from build123d import *

# Parameters (mm, degrees)
CROQUIS1_W              = 15.2
CROQUIS1_H              = 24.4
CROQUIS1_W_2            = 14
CROQUIS1_H_2            = 6.4
SALIENTE_EXTRUIR2_DEPTH = 8
SALIENTE_EXTRUIR4_START = 5
CROQUIS2_W              = 14
CROQUIS2_H              = 6.4
CROQUIS2_W_2            = 15.2
CROQUIS2_H_2            = 24.4
CROQUIS2_R              = 4
SALIENTE_EXTRUIR4_DEPTH = 5
CROQUIS3_R              = 4
CORTAR_EXTRUIR1_DEPTH   = 25
CROQUIS4_R              = 4
CORTAR_EXTRUIR2_DEPTH   = 30.02
CORTAR_EXTRUIR3_REACH   = 79.24
CROQUIS5_R              = 4.5


with BuildPart() as part:
    # Croquis1 → Saliente-Extruir2 (new body)
    with BuildSketch(Plane.XY):
        with BuildLine():
            Line((9.976185601, 29.499985584), (9.976185601, 16.499985584))
            Line((9.976185601, 16.499985584), (0.021811005, 16.499985584))
            ThreePointArc((0.021811005, 16.499985584), (-16.499996396, 0.010905505), (0, -16.5))
            Line((0, -16.5), (15, -16.5))
            Line((15, -16.5), (15, -29.5))
            Line((15, -29.5), (-14.857693224, -29.5))
            ThreePointArc((-14.857693224, -29.5), (-18.39322713, -28.035533906), (-19.857693224, -24.5))
            Line((-19.857693224, -24.5), (-19.857693224, -21.5))
            ThreePointArc((-19.857693224, -21.5), (-21.322159318, -17.964466094), (-24.857693224, -16.5))
            Line((-24.857693224, -16.5), (-56.53, -16.5))
            ThreePointArc((-56.53, -16.5), (-60.065533906, -15.035533906), (-61.53, -11.5))
            Line((-61.53, -11.5), (-61.53, 11.5))
            ThreePointArc((-61.53, 11.5), (-60.065533906, 15.035533906), (-56.53, 16.5))
            Line((-56.53, 16.5), (-24.857693224, 16.5))
            ThreePointArc((-24.857693224, 16.5), (-21.322159318, 17.964466094), (-19.857693224, 21.5))
            Line((-19.857693224, 21.5), (-19.857693224, 24.499985584))
            ThreePointArc((-19.857693224, 24.499985584), (-18.39322713, 28.03551949), (-14.857693224, 29.499985584))
            Line((-14.857693224, 29.499985584), (9.976185601, 29.499985584))
        make_face()
        with Locations((-49.43, 0)):
            Rectangle(CROQUIS1_W, CROQUIS1_H, mode=Mode.SUBTRACT)
        with Locations((-29, 0)):
            Rectangle(CROQUIS1_W_2, CROQUIS1_H_2, mode=Mode.SUBTRACT)
    extrude(amount=SALIENTE_EXTRUIR2_DEPTH)

    # Croquis2 → Saliente-Extruir4 (add)
    with BuildSketch(Plane(origin=(0, 0, 0), x_dir=(-1, 0, 0), z_dir=(0, 0, -1)).offset(SALIENTE_EXTRUIR4_START)):
        with BuildLine():
            Line((56.53, 16.5), (24.857693224, 16.5))
            ThreePointArc((24.857693224, 16.5), (21.322159318, 17.964466094), (19.857693224, 21.5))
            Line((19.857693224, 21.5), (19.857693224, 24.499985584))
            ThreePointArc((19.857693224, 24.499985584), (18.39322713, 28.03551949), (14.857693224, 29.499985584))
            Line((14.857693224, 29.499985584), (-9.976185601, 29.499985584))
            Line((-9.976185601, 29.499985584), (-9.976185601, 16.499985584))
            Line((-9.976185601, 16.499985584), (-0.021811005, 16.499985584))
            ThreePointArc((-0.021811005, 16.499985584), (8.607541842, 14.07693942), (14.696938457, 7.5))
            Line((14.696938457, 7.5), (0, 7.5))
            ThreePointArc((0, 7.5), (-5.303300859, 5.303300859), (-7.5, 0))
            Line((-7.5, 0), (-7.5, -16.5))
            Line((-7.5, -16.5), (-15, -16.5))
            Line((-15, -16.5), (-15, -29.5))
            Line((-15, -29.5), (14.857693224, -29.5))
            ThreePointArc((14.857693224, -29.5), (18.39322713, -28.035533906), (19.857693224, -24.5))
            Line((19.857693224, -24.5), (19.857693224, -21.5))
            ThreePointArc((19.857693224, -21.5), (21.322159318, -17.964466094), (24.857693224, -16.5))
            Line((24.857693224, -16.5), (56.53, -16.5))
            ThreePointArc((56.53, -16.5), (60.065533906, -15.035533906), (61.53, -11.5))
            Line((61.53, -11.5), (61.53, 11.5))
            ThreePointArc((61.53, 11.5), (60.065533906, 15.035533906), (56.53, 16.5))
        make_face()
        with Locations((29, 0)):
            Rectangle(CROQUIS2_W, CROQUIS2_H, mode=Mode.SUBTRACT)
        with Locations((49.43, 0)):
            Rectangle(CROQUIS2_W_2, CROQUIS2_H_2, mode=Mode.SUBTRACT)
        Circle(CROQUIS2_R, mode=Mode.SUBTRACT)
    extrude(amount=-SALIENTE_EXTRUIR4_DEPTH)

    # Croquis3 → Cortar-Extruir1 (cut)
    with BuildSketch(Plane(origin=(9.976185601, 0, 0), x_dir=(0, 0, -1), z_dir=(1, 0, 0))):
        with Locations(Location((-1.5, 23.151636707, 0), (0, 0, 90))):
            Circle(CROQUIS3_R)
    extrude(amount=-CORTAR_EXTRUIR1_DEPTH, mode=Mode.SUBTRACT)

    # Croquis4 → Cortar-Extruir2 (cut)
    with BuildSketch(Plane(origin=(15, 0, 0), x_dir=(0, 0, -1), z_dir=(1, 0, 0))):
        with Locations((-1.5, -22.848348878)):
            Circle(CROQUIS4_R)
    extrude(amount=-CORTAR_EXTRUIR2_DEPTH, mode=Mode.SUBTRACT)

    # Cortar-Extruir3: up to this face of the body (flat: up to its plane)
    cortar_extruir3_end = Plane(part.part.faces().sort_by_distance((-40.693846612, -16.5, 1.5))[0])
    # Croquis5 → Cortar-Extruir3 (cut, up to the picked face)
    with BuildSketch(Plane(origin=(0, 16.5, 0), x_dir=(1, 0, 0), z_dir=(0, 1, 0)), mode=Mode.PRIVATE) as cortar_extruir3_sk1:
        with Locations(Location((-49.43, -1.5, 0), (0, 0, 180))):
            Circle(CROQUIS5_R)
    cortar_extruir3_tool1 = split(extrude(cortar_extruir3_sk1.sketch, amount=-CORTAR_EXTRUIR3_REACH, mode=Mode.PRIVATE), bisect_by=cortar_extruir3_end, keep=Keep.BOTH, mode=Mode.PRIVATE)
    # Croquis5 → Cortar-Extruir3 (cut, up to the picked face)
    with BuildSketch(Plane(origin=(0, 16.5, 0), x_dir=(1, 0, 0), z_dir=(0, 1, 0)), mode=Mode.PRIVATE) as cortar_extruir3_sk2:
        with Locations(Location((-29, -1.5, 0), (0, 0, 270))):
            Circle(CROQUIS5_R)
    cortar_extruir3_tool2 = split(extrude(cortar_extruir3_sk2.sketch, amount=-CORTAR_EXTRUIR3_REACH, mode=Mode.PRIVATE), bisect_by=cortar_extruir3_end, keep=Keep.BOTH, mode=Mode.PRIVATE)
    add(cortar_extruir3_tool1.solids().sort_by(Axis((-49.43, 16.5, 1.5), (0, -1, 0)))[0], mode=Mode.SUBTRACT)
    add(cortar_extruir3_tool2.solids().sort_by(Axis((-29, 16.5, 1.5), (0, -1, 0)))[0], mode=Mode.SUBTRACT)


solid = part.part
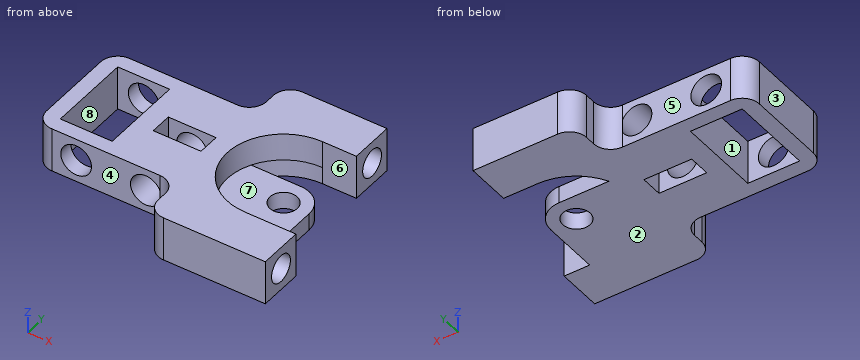
Verification items for the finished model (mm, model axes). Face numbers are marked on the shaded views. A direction names the side the tool comes from. Coordinates: 2 decimals unless noted, no trailing zeros. Loops run counter-clockwise (first coordinate to the right, second up) from the corner with the lowest first, then second, coordinate; pieces in that order, holes last. Notation, with made-up numbers: (82.25, 78) -> (131.25, 78) arc R12 cw to (131.25, 95) -> close; hole circle Ø5 at (26, 81.5). An arc over 180 degrees is marked (long way). Write each question's results on one line, items separated by ' | '.
Item 1: Mould release check, pull along X, two halves, no side actions. Record for the marked faces 1, 2 and 3: +X half, -X half, draft (parallel to the pull), parting line (faces both ways), or undercut.
Found:
face 1: undercut | face 2: draft | face 3: -X half
Item 2: Section check B-B, the plane y = -9. Enter the section's corners in (x, z).
Found:
outline: (-61.53, -5) -> (-57.03, -5) -> (-57.03, 8) -> (-61.53, 8) -> close; (-41.83, -5) -> (7.5, -5) -> (7.5, 0) -> (-13.83, 0) -> (-13.83, 8) -> (-41.83, 8) -> close; hole circle Ø9 at (-29, 1.5)
Item 3: Section check A-A, the plane x = -29. Enter the section's corners in (y, z), plus the area to 3 significant figures.
Found:
outline: (-16.5, -5) -> (-3.2, -5) -> (-3.2, -3) -> (-16.5, -3) -> close; (-16.5, 6) -> (-3.2, 6) -> (-3.2, 8) -> (-16.5, 8) -> close; (3.2, -5) -> (16.5, -5) -> (16.5, -3) -> (3.2, -3) -> close; (3.2, 6) -> (16.5, 6) -> (16.5, 8) -> (3.2, 8) -> close | area: 106 mm2
Item 4: Section check D-D, the plane x = -49.43. Enter the section's corners in (y, z).
Found:
outline: (-16.5, -5) -> (-12.2, -5) -> (-12.2, -3) -> (-16.5, -3) -> close; (-16.5, 6) -> (-12.2, 6) -> (-12.2, 8) -> (-16.5, 8) -> close; (12.2, -5) -> (16.5, -5) -> (16.5, -3) -> (12.2, -3) -> close; (12.2, 6) -> (16.5, 6) -> (16.5, 8) -> (12.2, 8) -> close
Item 5: Tool access check on the marked faces 4, 5, 6, 7 and 8. Record the directions out of +Z, -Z, +X, -X, +Y, -Y that give a thin tool (end or side, any length) a straight path to the whole face; none if there is none.
Found:
face 4: +Z, -Z, -X, -Y | face 5: +Z, -Z, -X, +Y | face 6: +Z, -Z, +X | face 7: +Z, +X | face 8: +Z, -Z
Item 6: Section check C-C, the plane z = -4. Count the separate pieces of the cut face and the enclosed holes in it, plus the area to 3 significant figures.
Found:
separate pieces: 1 | enclosed holes: 3 | area: 2,420 mm2
Item 7: Material ranges on L1, parallel to Z at x = -29, y = 7; L2, parallel to X at y = 3, z = 2.75; L3, parallel to X at y = -11, z = 1.5, recorded low to high.
Found:
L1: z = -5 to -3, 6 to 8 | L2: x = -61.53 to -57.03, -41.83 to -36, -22 to -16.22 | L3: x = -61.53 to -57.03, -41.83 to -33.5, -24.5 to -12.3
Item 8: Gauge pin test, flat ends, axial feed: pin 1 (6.5 mm diameter, centred on y = 26, z = -0.5, fed in from +X); pin 2 (2 mm diameter, centred on x = 2.5, y = -9.5, fed in from +Z); pin 3 (3 mm diameter, centred on x = -45.5, z = 3, fed in from +Y). Record the tip position at first contact, or that the pin passes through.
Found:
pin 1: stops at x = 9.98 | pin 2: stops at z = 0 | pin 3: stops at y = 16.5
